Can you work these out from the model? Positions are in its coordinate system, mm. Face numbers are marked on the shaded views. A direction names the side the tool comes from. Give positions to 0.01 mm unless a question says otherwise; leave off trailing zeros. Order: outer loops, then holes, each group sorted by start corner. A loop starts at its lowest first (then second) coordinate and runs counter-clockwise, first axis right, second up. Notation, with made-up numbers: (-32.5, 48) - (21.5, 48) arc R24 ccw to (21.5, 65) - close; hole circle Ø9 at (65, 86.25). An arc over 180 degrees is marked (long way). Use one line per item in the form item = value. Start each with the question number.
1) Suppose I cut it at A-A, the plane x = 318.5. Write out the boundary of the cut face in (y, z), and give its area (3 significant figures).
2) Suppose I cut it at B-B, the plane y = -489. Write out the boundary of the cut face in (x, z).
3) Please list where these lines run through material, in increasing order: probe 1 along Y at (x, z) = (68, 867); probe 2 along X at (y, z) = (-286, 503); probe 3 along Z at (x, y) = (134.5, -371).
4) Which directions (+Z, -Z, +X, -X, +Y, -Y) give clear straight access to the entire face, cutting with the end or side of a thin tool? Please do the marked faces 1 and 2.
5) For pin 1 (1.5 mm diameter, centred on y = -326, z = -215.5, fed in from +X); pin 2 (1 mm diameter, centred on x = 218, y = -366.5, fed in from +Z); pin 3 (1 mm diameter, centred on x = 348.5, z = -35.5, fed in from -Y), each with a flat end and sliding along its axis, tell me the tip position at first contact or that it passes through.
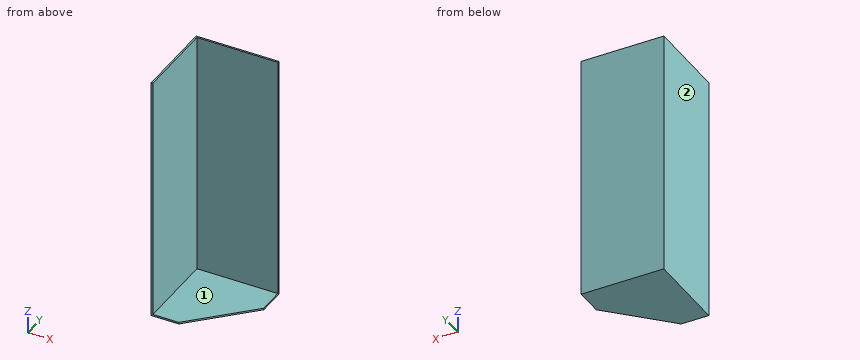
```python
from build123d import *

# Parameters (mm, degrees)
F0_W     = 609.6
F0_H     = 1828.8
F1_DEPTH = 12.7
F4_W     = 596.9
F4_H     = 596.9
F5_DEPTH = 12.7
F6_SIZE  = 406.4


# Not quite as in the source:
# - a feature of the source that left no trace in its solid (it failed there, or was rolled back) is left out
# - a pattern or mirror of a feature is missing from the dataset's text; its kind, count and spacing are read off the source's solid


with BuildPart() as f1:
    # F0 (on Front) → F1 (new body)
    with BuildSketch(Plane.XZ):
        with Locations((304.8, 85.8015570831)):
            Rectangle(F0_W, F0_H)
    extrude(amount=F1_DEPTH)

    # F1_copies: F1 across plane


with BuildPart() as f1_1:
    add(f1.part)
    add(f1.part.mirror(Plane(origin=(0, 0, 0), x_dir=(0.7071067812, -0.7071067812, 0), z_dir=(-0.7071067812, -0.7071067812, 0))))

    # F4 (on face) → F5 (join)
    with BuildSketch(Plane(origin=(0, 0, -828.5984429169), x_dir=(1, 0, 0), z_dir=(0, 0, -1))):
        with Locations((311.15, 311.15)):
            Rectangle(F4_W, F4_H)
    extrude(amount=-F5_DEPTH)

    # F6
    f6_edges = [f1_1.edges().sort_by_distance(p)[0] for p in [
        (609.6, -609.6, -822.248443),
    ]]
    chamfer(f6_edges, length=F6_SIZE)


solid = f1_1.part
```
Result sheet:
q1.outline = (-494.3, -828.6) - (0, -828.6) - (0, 1000.2) - (-12.7, 1000.2) - (-12.7, -815.9) - (-494.3, -815.9) - close
q1.area = 29,300 mm²
q2.outline = (0, -828.6) - (323.8, -828.6) - (323.8, -815.9) - (12.7, -815.9) - (12.7, 1000.2) - (0, 1000.2) - close
q3.probe_1 = -12.7 to 0
q3.probe_2 = 0 to 12.7
q3.probe_3 = -828.6 to -815.9
q4.face_1 = +Z, +X, -Y
q4.face_2 = +Z, -Z, -X, +Y, -Y
q5.pin_1 = 12.7
q5.pin_2 = -815.9
q5.pin_3 = -12.7
